Job drawing, mm, ordinate dimensions from the low corner. One solid piece. A direction names the side the tool comes from. Coordinates: 2 decimals unless noted, no trailing zeros. Write each loop counter-clockwise with the first axis right and the second up, starting at its lowest first coordinate (ties: lowest second). Pieces come first, ordered by that corner, then holes. Notation, with made-up numbers: (12, 24.5) - (45, 24.5) arc R12 cw to (45, 35.5) - close; hole circle Ø2 at (69, 38.25). An arc over 180 degrees is marked (long way). Put each result on its own line as item: value. Start each with the question number.
1. Saw through at B-B, the plane y = 6.5. Write the cut outline in (x, z), plus the area to 3 significant figures.
2. Saw through at D-D, the plane z = 15. Write the cut outline in (x, y), plus the area to 3 significant figures.
3. Pull direction X, two halves, no side cores. Call the marked faces 1 and 2: released by +X, released by -X, zero draft, split by the parting line, or undercut.
4. Saw through at A-A, the plane x = 27.65. Write the cut outline in (y, z), plus the area to 3 significant figures.
5. Saw through at C-C, the plane x = 15.45. Write the cut outline in (y, z).
6. Which spindle directions (+Z, -Z, +X, -X, +Y, -Y) get a long thin tool onto all of the face, cutting with end or side? Do the marked faces 3 and 4. Say none if no direction does.
7. Drop flat-ended pins along their axis: P1, Ø2, axis at y = 1.5, z = 6.5, coming from the +X side; P2, Ø5, axis at x = 18, z = 14, coming from the -Y side; P3, Ø2, axis at x = 8, y = 7, coming from the +Z side; P4, Ø1.8, axis at x = 10.95, z = 10, coming from the +Y side. Give the stop position or say it passes through.
8. Drill centre lines: L1, parallel to Z at x = 15.45, y = 4.75; L2, parallel to X at y = 5.25, z = 11; L3, parallel to Z at x = 27.65, y = 6. Where is each one in solid material? Low to high. Write a range as from..to.
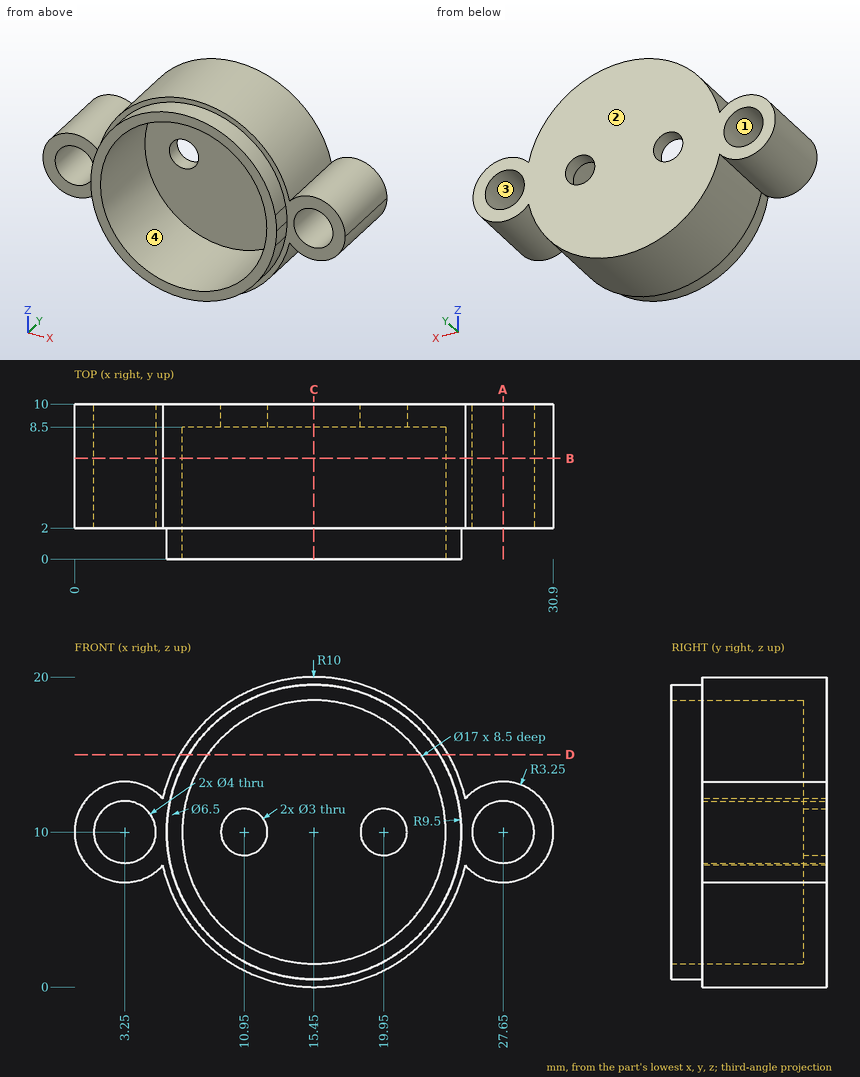
Final values:
1. outline: (5.68, 7.85) arc R10 ccw to (25.22, 7.85) arc R3.25 ccw (long way) to (25.22, 12.15) arc R10 ccw to (5.68, 12.15) arc R3.25 ccw (long way) to start; hole circle Ø4 at (3.25, 10); hole circle Ø17 at (15.45, 10); hole circle Ø4 at (27.65, 10)
1. area: 122 mm²
2. outline: (6.79, 2) - (7.37, 2) - (7.37, 0) - (8.58, 0) - (8.58, 8.5) - (22.32, 8.5) - (22.32, 0) - (23.53, 0) - (23.53, 2) - (24.11, 2) - (24.11, 10) - (6.79, 10) - close
2. area: 54.0 mm²
3. face 1: undercut
3. face 2: zero draft
4. outline: (2, 6.75) - (10, 6.75) - (10, 8) - (2, 8) - close; (2, 12) - (10, 12) - (10, 13.25) - (2, 13.25) - close
4. area: 20.0 mm²
5. outline: (0, 0.5) - (2, 0.5) - (2, 0) - (10, 0) - (10, 20) - (2, 20) - (2, 19.5) - (0, 19.5) - (0, 18.5) - (8.5, 18.5) - (8.5, 1.5) - (0, 1.5) - close
6. face 3: +Y, -Y
6. face 4: -Y
7. P1: stops at x = 29.55
7. P2: stops at y = 8.5
7. P3: stops at z = 17.64
7. P4: passes through
8. L1: z = 0..1.5, 18.5..20
8. L2: x = 0.16..1.52, 4.98..7.01, 23.89..25.92, 29.38..30.74
8. L3: z = 6.75..8, 12..13.25
